from build123d import *

# Parameters (mm, degrees)
F0_W      = 590
F0_H      = 590
F1_DEPTH  = 22
F7_DEPTH  = 590.001
F8_DEPTH  = 590.001
F9_DEPTH  = 590.001
F10_DEPTH = 590.001
F11_W     = 50
F11_H     = 50
F12_DEPTH = 10


with BuildPart() as f1:
    # F0 (on Top) → F1 (new body)
    with BuildSketch(Plane.XY):
        with Locations((295, 295)):
            Rectangle(F0_W, F0_H)
    extrude(amount=F1_DEPTH)

    # F3 (on face) → F7 (cut, through all)
    with BuildSketch(Plane.XZ):
        Polygon((0, 14.5), (0, 0), (12.1669, 0), align=None)
    extrude(amount=-F7_DEPTH, mode=Mode.SUBTRACT)

    # F4 (on face) → F8 (cut, through all)
    with BuildSketch(Plane.YZ.offset(590)):
        Polygon((0, 14.5), (0, 0), (12.1669, 0), align=None)
    extrude(amount=-F8_DEPTH, mode=Mode.SUBTRACT)

    # F5 (on face) → F9 (cut, through all)
    with BuildSketch(Plane(origin=(0, 0, 0), x_dir=(0, -1, 0), z_dir=(-1, 0, 0))):
        Polygon((-590, 14.5), (-590, 0), (-577.8331, 0), align=None)
    extrude(amount=-F9_DEPTH, mode=Mode.SUBTRACT)

    # F6 (on face) → F10 (cut, through all)
    with BuildSketch(Plane(origin=(0, 590, 0), x_dir=(-1, 0, 0), z_dir=(0, 1, 0))):
        Polygon((-590, 14.5), (-590, 0), (-577.8331, 0), align=None)
    extrude(amount=-F10_DEPTH, mode=Mode.SUBTRACT)

    # F11 (on face) → F12 (cut)
    with BuildSketch(Plane(origin=(0, 0, 0), x_dir=(1, 0, 0), z_dir=(0, 0, -1))):
        with Locations((44.9669, -44.9669)):
            Rectangle(F11_W, F11_H)
        with Locations((545.0331, -44.9669)):
            Rectangle(F11_W, F11_H)
        with Locations((44.9669, -545.0331)):
            Rectangle(F11_W, F11_H)
        with Locations((545.0331, -545.0331)):
            Rectangle(F11_W, F11_H)
    extrude(amount=-F12_DEPTH, mode=Mode.SUBTRACT)


solid = f1.part
Could you check a few things on this model? Use its own coordinates, in mm. A direction names the side the tool comes from. Give positions to 0.01 mm unless a question says otherwise; leave off trailing zeros. Order: outer loops, then holes, each group sorted by start corner. A loop starts at its lowest first (then second) coordinate and runs counter-clockwise, first axis right, second up.
1. I need wall thicknesses on L1, parallel to X at y = 35, z = 9.5; L2, parallel to X at y = 452, z = 3.5; L3, parallel to X at y = 490, z = 12.75. Which ranges of each line are inside material? Lowest first, please.
Answers below:
L1: x = 4.2 to 19.97, 69.97 to 520.03, 570.03 to 585.8
L2: x = 9.23 to 580.77
L3: x = 1.47 to 588.53
2. Suppose I cut it at A-A (y = 542). Write out the boundary of the cut face in (x, z), plus the area to 3 significant figures.
Answers below:
outline: (0, 14.5) - (12.17, 0) - (19.97, 0) - (19.97, 10) - (69.97, 10) - (69.97, 0) - (520.03, 0) - (520.03, 10) - (570.03, 10) - (570.03, 0) - (577.83, 0) - (590, 14.5) - (590, 22) - (0, 22) - close
area: 11,800 mm2
3. Thinking about a two-plate mould opening in X: for faces 1 (the flat face through (583.831, 299.13, 7.149)), 2 (the flat face through (6.169, 290.87, 7.148)), 3 (the flat face through (45, 45, 10)), 4 (the flat face through (291, 299, 22)), which applies, +X half, -X half, draft (parallel to the pull), parting line (faces both ways), or undercut?
Answers below:
face 1: +X half
face 2: -X half
face 3: undercut
face 4: draft
4. Suppose I cut it at C-C (z = 5.25). Write out the boundary of the cut face in (x, y).
Answers below:
outline: (7.76, 7.76) - (582.24, 7.76) - (582.24, 582.24) - (7.76, 582.24) - close; hole (19.97, 19.97) - (69.97, 19.97) - (69.97, 69.97) - (19.97, 69.97) - close; hole (19.97, 520.03) - (69.97, 520.03) - (69.97, 570.03) - (19.97, 570.03) - close; hole (520.03, 19.97) - (570.03, 19.97) - (570.03, 69.97) - (520.03, 69.97) - close; hole (520.03, 520.03) - (570.03, 520.03) - (570.03, 570.03) - (520.03, 570.03) - close
5. For pin 1 (6 mm diameter, centred on y = 271, z = 6, fed in from -X); pin 2 (2 mm diameter, centred on y = 478.5, z = 10, fed in from +X); pin 3 (8 mm diameter, centred on x = 53.5, z = 3, fed in from +Y), each with a flat end and sliding along its axis, tell me the tip position at first contact or that it passes through.
Answers below:
pin 1: stops at x = 4.62
pin 2: stops at x = 587.06
pin 3: stops at y = 583.71
6. Which directions (+Z, -Z, +X, -X, +Y, -Y) give clear straight access to the entire face, cutting with the end or side of a thin tool? Please do faces 5 (the flat face through (45, 545, 10)), 6 (the flat face through (291, 299, 0)).
Answers below:
face 5: -Z
face 6: -Z, +X, -X, +Y, -Y
